```python
from build123d import *

# Parameters (mm, degrees)
F1_DEPTH = 15
F3_DEPTH = 5


with BuildPart() as f1:
    # F0 (on Right) → F1 (new body)
    with BuildSketch(Plane.YZ):
        Polygon((-3.5355339059, 3.5355339059), (0, 0), (15, 0), (15, 19.7983665757), (4.7861494543, 19.7983665757), (1.4644660941, 8.5355339059), (-3.5355339059, 8.5355339059), align=None)
    extrude(amount=-F1_DEPTH)

    # F2 (on face) → F3 (cut)
    with BuildSketch(Plane(origin=(-15, 0, 0), x_dir=(0, -1, 0), z_dir=(-1, 0, 0))):
        Polygon((-4.7861494543, 19.7983665757), (-15, 19.7983665757), (-1.4644660941, 8.5355339059), align=None)
    extrude(amount=-F3_DEPTH, mode=Mode.SUBTRACT)

    # F6: F1 across plane


with BuildPart() as f1_1:
    add(f1.part)
    add(f1.part.mirror(Plane.YZ.offset(-15)))


solid = f1_1.part
```
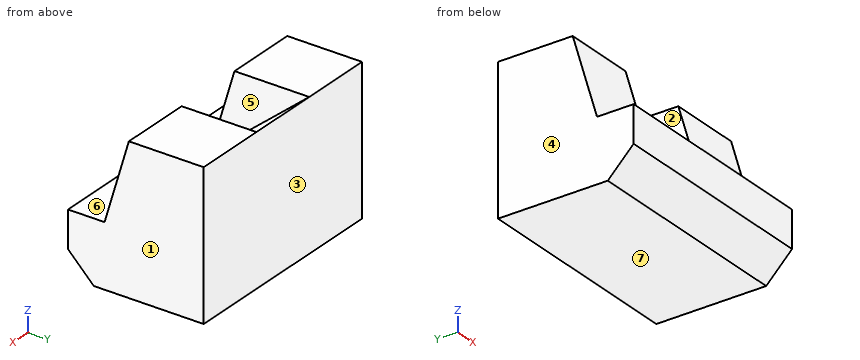
For this review, take the finished solid that the model builds, in its own axes (mm). Face numbers are marked on the shaded views. A direction names the side the tool comes from. Give positions to 0.01 mm unless a question says otherwise; leave off trailing zeros. Order: outer loops, then holes, each group sorted by start corner. A loop starts at its lowest first (then second) coordinate and runs counter-clockwise, first axis right, second up.
1) Take a section at A-A (x = -18.5). Give the boundary of the cut face in (y, z), then the cut area to 3 significant figures.
2) Take a section at B-B (z = 11.5). Give the boundary of the cut face in (x, y), then the cut area to 3 significant figures.
3) Wall thickness on line 1 (Y direction, x = -27.25, z = 17.5); line 2 (Z direction, x = -12, y = -1); line 3 (Z direction, x = -17, y = 8): over which ranges is each line inside the solid? List them lowest first.
4) For the marked faces 5, 6 and 7, list the 3-axis set-ups (+Z, -Z, +X, -X, +Y, -Y) from which the entire face can be reached by the end or side of a thin tool; tool diameter is ignored.
5) Take a section at C-C (y = 3). Give the boundary of the cut face in (x, z).
6) The part is to be moulded in two halves that separate along X. For the marked faces 1, 2, 3 and 4, say which applies: released by +X, released by -X, zero draft, split by the parting line, or undercut.
7) Take a section at D-D (x = -25.25). Give the boundary of the cut face in (y, z).
8) Insertion check: pin 1 (1.5 mm diameter, centred on y = 13, z = 10, fed in from +X). The pin has a flat end and moves straight along its axis. Give the tip position at first contact, or say it passes through.
Derived:
1. outline: (-3.54, 3.54) - (0, 0) - (15, 0) - (15, 19.8) - (1.46, 8.54) - (-3.54, 8.54) - close
1. area: 228 mm2
2. outline: (-30, 2.34) - (-20, 2.34) - (-20, 5.03) - (-10, 5.03) - (-10, 2.34) - (0, 2.34) - (0, 15) - (-30, 15) - close
2. area: 353 mm2
3. line 1: y = 4.11 to 15
3. line 2: z = 1 to 8.54
3. line 3: z = 0 to 13.97
4. face 5: +Z, -Y
4. face 6: +Z, +X, -X, -Y
4. face 7: -Z, +X, -X, +Y, -Y
5. outline: (-30, 0) - (0, 0) - (0, 13.74) - (-10, 13.74) - (-10, 9.81) - (-20, 9.81) - (-20, 13.74) - (-30, 13.74) - close
6. face 1: released by +X
6. face 2: undercut
6. face 3: zero draft
6. face 4: released by -X
7. outline: (-3.54, 3.54) - (0, 0) - (15, 0) - (15, 19.8) - (4.79, 19.8) - (1.46, 8.54) - (-3.54, 8.54) - close
8. pin 1: stops at x = 0
